Build history of the part. All positions in model axes, mm. Give positions to 0.01 mm unless a question says otherwise; leave off trailing zeros. Order: outer loops, then holes, each group sorted by start corner. A loop starts at its lowest first (then second) coordinate and runs counter-clockwise, first axis right, second up. Notation, with made-up numbers: M 61,65 L 115,65 A10 cw 115,74 Z; hole C -27,39 d11. An arc over 180 degrees is marked long. One line per item, written item: value.
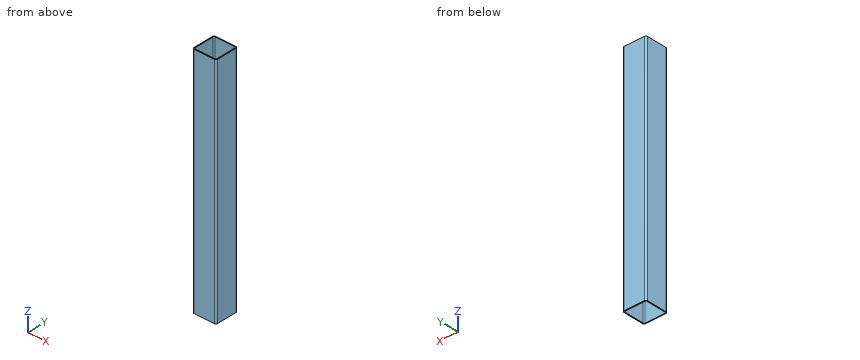
Autodesk Inventor part; units mm, degrees
ref_plane "Start Plane" through (0, 0, 0) normal (0, 0, 1) x (1, 0, 0)
ref_plane "End Plane" through (0, 0, 792) normal (0, 0, 1) x (1, 0, 0)
ref_plane "YZ Plane" through (0, 0, 0) normal (1, 0, 0) x (0, 1, 0)
ref_plane "Start Plane" through (0, 0, 0) normal (0, 0, 1) x (1, 0, 0)
ref_plane "End Plane" through (0, 0, 792) normal (0, 0, 1) x (1, 0, 0)
sketch "Sketch" plane through (0, 0, 0) normal (0, 0, 1) x (1, 0, 0)
  line L0 (-40, -34) -> (-40, 34)
  line L1 (-34, 40) -> (34, 40)
  line L2 (40, 34) -> (40, -34)
  line L3 (34, -40) -> (-34, -40)
  arc A0 (-40, -34) -> (-34, -40) centre (-34, -34) ccw
  arc A1 (40, 34) -> (34, 40) centre (34, 34) ccw
  arc A2 (-34, 40) -> (-40, 34) centre (-34, 34) ccw
  arc A3 (34, -40) -> (40, -34) centre (34, -34) ccw
  arc A4 (-34, 37) -> (-37, 34) centre (-34, 34) ccw
  line L4 (-34, 37) -> (34, 37)
  arc A5 (37, 34) -> (34, 37) centre (34, 34) ccw
  line L5 (37, 34) -> (37, -34)
  arc A6 (34, -37) -> (37, -34) centre (34, -34) ccw
  line L6 (34, -37) -> (-34, -37)
  arc A7 (-37, -34) -> (-34, -37) centre (-34, -34) ccw
  line L7 (-37, -34) -> (-37, 34)
  line L8 (0, 57.7397) -> (0, -57.7397) construction
  line L9 (-57.7397, 0) -> (57.7397, 0) construction
  dimension "d7" = 6
  dimension "d9" = 80
  dimension "d11" = 80
  dimension "d12" = 3
  dimension "d15" = 40
  dimension "d16" = 40
extrude "Body" add sketch "Sketch" along normal blind 792 from surface at 0
sketch "Sketch3" plane through (0, 0, 0) normal (0, 0, 1) x (1, 0, 0)
  line L0 (0, 0) -> (10, 0)
ref_plane "Work Plane3" through (0, 0, 0) normal (0, -1, 0) x (1, 0, 0)
sketch "Sketch4" plane through (0, 0, 0) normal (0, -1, 0) x (1, 0, 0)
  line L0 (-2, 0) -> (12, 0)
  line L1 (-2, 792) -> (12, 792)
  dimension "d18" = 792
equation "\"d7\" = G_IR"
equation "\"d9\" = G_W"
equation "\"d11\" = G_H"
equation "\"d12\" = G_T"
equation "\"d15\" = 0.5 * d9"
equation "\"d16\" = 0.5 * d11"
equation "\"d3\" = G_L"
equation "\"G_W\" = 80"
equation "\"G_H\" = 80"
equation "\"G_T\" = 3"
equation "\"G_IR\" = 6"
equation "\"G_L\" = d18"
equation "\"G_OFFSET_START\" = 0"
equation "\"G_OFFSET_END\" = 0"
equation "\"d14\" = G_OFFSET_END + B_L"
equation "\"B_L\" = 792"
properties part number "ISO 10799-2 - 80x80x3 - 792" material "Steel, Mild"
1) Drill centre line: probe 1 along Y at (x, z) = (-27, 679). Where is it in solid material? Low to high. Write a range as from..to.
Check values:
probe 1: -40..-37, 37..40
2) Saw through at B-B, the plane z = 175. Write the cut outline in (x, y), then the cut area to 3 significant figures.
Check values:
outline: M -40,-34 A6 ccw -34,-40 L 34,-40 A6 ccw 40,-34 L 40,34 A6 ccw 34,40 L -34,40 A6 ccw -40,34 Z; hole M -37,-34 A3 ccw -34,-37 L 34,-37 A3 ccw 37,-34 L 37,34 A3 ccw 34,37 L -34,37 A3 ccw -37,34 Z
area: 901 mm^2
3) Saw through at A-A, the plane x = 6. Write the cut outline in (y, z), then the cut area to 3 significant figures.
Check values:
outline: M -40,0 L -37,0 L -37,792 L -40,792 Z; M 37,0 L 40,0 L 40,792 L 37,792 Z
area: 4,750 mm^2
